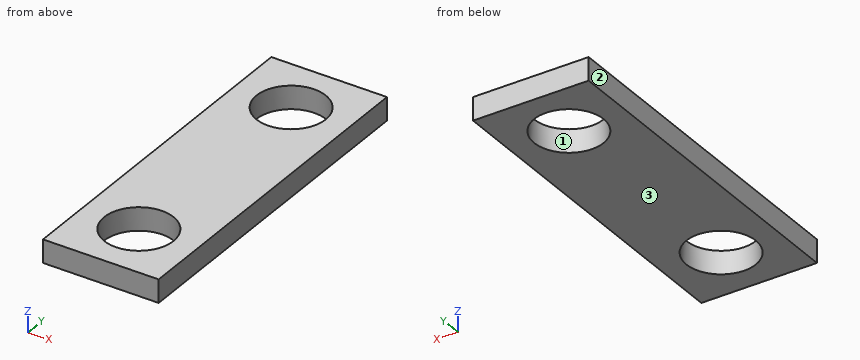
Autodesk Inventor part; units mm, degrees
ref_plane "YZ Plane" through (0, 0, 0) normal (1, 0, 0) x (0, 1, 0)
ref_plane "XZ Plane" through (0, 0, 0) normal (0, 1, 0) x (-1, 0, 0)
ref_plane "XY Plane" through (0, 0, 0) normal (0, 0, 1) x (1, 0, 0)
sketch "スケッチ1" plane through (0, 0, 0) normal (0, 0, 1) x (1, 0, 0)
  line L0 (0, 0) -> (10, 0)
  line L1 (10, 0) -> (10, 30)
  line L2 (10, 30) -> (0, 30)
  line L3 (0, 30) -> (0, 0)
  dimension "d0" = 10
  dimension "d1" = 30
extrude "押し出し1" add sketch "スケッチ1" along normal blind 2
sketch "スケッチ2" plane through (0, 0, 2) normal (0, 0, 1) x (1, 0, 0)
  line L0 (0, 0) -> (10, 0)
  line L1 (10, 30) -> (0, 30)
  line L2 (0, 30) -> (0, 0)
  point P0 (5, 5)
  point P1 (5, 25)
  dimension "d4" = 5
  dimension "d12" = 5
  dimension "d13" = 5
hole "穴1" at (5, 5, 2) at (5, 25, 2) direction (0, 0, -1) diameter 6 end through all
properties part number "指先"
The listing builds one solid part. Answer for the finished solid, in the listing's coordinates (mm). Face numbers are marked on the shaded views. Coordinates: 2 decimals unless noted, no trailing zeros. Write each loop counter-clockwise with the first axis right and the second up, starting at its lowest first coordinate (ties: lowest second). Pieces come first, ordered by that corner, then holes. Notation, with made-up numbers: M 76,27 L 107,27 A28 ccw 107,65 Z; hole C 62,31 d1. An arc over 180 degrees is marked long. Put each result on its own line as item: value. Start each with the question number.
1. For a pull along X with two mould halves and no side action, classify the marked faces 1, 2 and 3 as pulls with the +X half, pulls with the -X half, needs draft (parallel to the pull), parting line crosses it, or undercut.
2. A flat-ended cylindrical pin translates along its axis: P1, Ø5, axis at x = 5, y = 5, coming from the +Z side. Find the tip coordinate at first contact, or state that the pin passes through.
3. Consider line 1 (Y direction, x = 5, z = 1.5); line 2 (Y direction, x = 3.5, z = 1.1); line 3 (X direction, y = 25, z = 1.1). Determine where each line is inside the solid, lowest interval first. Write a range as from..to.
4. A cutting plane is placed at A-A on x = 5. Write down the section's boundary in (y, z), then the cut area to 3 significant figures.
5. A cutting plane is placed at D-D on x = 6.25. Write down the section's boundary in (y, z), then the cut area to 3 significant figures.
6. A cutting plane is placed at C-C on z = 1.35. Write down the section's boundary in (x, y).
7. A cutting plane is placed at B-B on y = 25. Write down the section's boundary in (x, z).
Resolved:
1. face 1: undercut
1. face 2: pulls with the -X half
1. face 3: needs draft
2. P1: passes through
3. line 1: y = 0..2, 8..22, 28..30
3. line 2: y = 0..2.4, 7.6..22.4, 27.6..30
3. line 3: x = 0..2, 8..10
4. outline: M 0,0 L 2,0 L 2,2 L 0,2 Z; M 8,0 L 22,0 L 22,2 L 8,2 Z; M 28,0 L 30,0 L 30,2 L 28,2 Z
4. area: 36.0 mm2
5. outline: M 0,0 L 2.27,0 L 2.27,2 L 0,2 Z; M 7.73,0 L 22.27,0 L 22.27,2 L 7.73,2 Z; M 27.73,0 L 30,0 L 30,2 L 27.73,2 Z
5. area: 38.2 mm2
6. outline: M 0,0 L 10,0 L 10,30 L 0,30 Z; hole C 5,5 d6; hole C 5,25 d6
7. outline: M 0,0 L 2,0 L 2,2 L 0,2 Z; M 8,0 L 10,0 L 10,2 L 8,2 Z
